Source: CAD feature listing. Evaluate the final solid. Frame: model axes, mm. A direction names the side the tool comes from. Give positions to 0.01 mm unless a question says otherwise; leave off trailing zeros. Order: outer loops, then holes, each group sorted by start corner. A loop starts at its lowest first (then second) coordinate and runs counter-clockwise, first axis right, second up. Notation, with made-up numbers: (66, -23.75) - (103, -23.75) arc R17 cw to (103, 2.25) - close; hole circle Ø10 at (4, 41). An arc over 180 degrees is marked (long way). Use CSV: the item, a comma, the result in double quotes.
```python
from build123d import *

# Parameters (mm, degrees)
BOSS_EXTRUDE1_DEPTH = 10
CUT_EXTRUDE23_DEPTH = 10


with BuildPart() as part:
    # Sketch1 → Boss-Extrude1 (new body)
    with BuildSketch(Plane.XY):
        with BuildLine():
            Line((-50, 60), (50, 60))
            ThreePointArc((50, 60), (57.071067812, 57.071067812), (60, 50))
            Line((60, 50), (60, -50))
            ThreePointArc((60, -50), (57.071067812, -57.071067812), (50, -60))
            Line((50, -60), (-50, -60))
            ThreePointArc((-50, -60), (-57.071067812, -57.071067812), (-60, -50))
            Line((-60, -50), (-60, 50))
            ThreePointArc((-60, 50), (-57.071067812, 57.071067812), (-50, 60))
        make_face()
    extrude(amount=BOSS_EXTRUDE1_DEPTH)

    # Sketch2 → Cut-Extrude23 (cut)
    with BuildSketch(Plane.XY.offset(10)):
        with BuildLine():
            Line((-8.75, 50), (8.75, 50))
            Line((8.75, 50), (8.75, -14.7265625))
            add(Edge.make_bspline(
                [(8.75, -14.7265625), (8.743583975, -15.963662149), (8.731221561, -18.347308928), (8.60745187, -21.778880386), (8.440093422, -24.925119282), (8.199081109, -27.780984325), (7.841111838, -30.346337414), (7.435999316, -32.627578869), (6.989047753, -34.634004111), (6.23403689, -36.879506107), (5.061904404, -39.366144137), (3.293123023, -42.05206658), (1.090424054, -44.385675502), (-1.446357574, -46.412684578), (-4.338596124, -48.017692334), (-7.51966122, -49.177796237), (-10.979383755, -49.870850344), (-13.375676653, -49.956106859), (-14.609375, -50)],
                knots=[0, 0, 0, 0, 1.22248561, 2.355488409, 3.392943897, 4.335991845, 5.186735882, 5.951517034, 6.625683685, 7.215700098, 8.28923535, 9.333114649, 10.380102123, 11.447198135, 12.530158036, 13.633358744, 14.781567393, 16, 16, 16, 16], degree=3))
            add(Edge.make_bspline(
                [(-14.609375, -50), (-15.894776413, -49.960205451), (-18.430089946, -49.88171506), (-22.148388349, -49.2131785), (-25.722137923, -48.141313235), (-29.13284997, -46.591524706), (-32.427252281, -44.650205179), (-35.545554474, -42.242187263), (-38.552862415, -39.442154155), (-40.33561292, -37.293479019), (-41.25, -36.19140625)],
                knots=[0, 0, 0, 0, 0.990984786, 1.954608977, 2.90473533, 3.862451285, 4.837525908, 5.848096122, 6.896271184, 8, 8, 8, 8], degree=3))
            Line((-41.25, -36.19140625), (-28.0078125, -23.9453125))
            add(Edge.make_bspline(
                [(-28.0078125, -23.9453125), (-27.314466509, -24.729291012), (-26.01702976, -26.196325573), (-24.061830829, -28.109374669), (-22.298136041, -29.64628881), (-20.635555645, -30.75487882), (-19.06661841, -31.53631102), (-17.557567552, -32.099198603), (-16.061363785, -32.417824942), (-15.072925956, -32.473022924), (-14.58984375, -32.5)],
                knots=[0, 0, 0, 0, 1.529509877, 2.862124173, 3.996688592, 4.944357383, 5.774364335, 6.554177287, 7.293378699, 8, 8, 8, 8], degree=3))
            add(Edge.make_bspline(
                [(-14.58984375, -32.5), (-14.122273945, -32.475616988), (-13.223290925, -32.428736471), (-11.987154797, -31.907600104), (-10.945012492, -31.089394098), (-10.25892751, -30.148760123), (-9.821709802, -29.187178965), (-9.548527937, -28.257662954), (-9.289277875, -27.143425185), (-9.081572506, -25.845024103), (-8.924629957, -24.345523841), (-8.846405442, -22.663128248), (-8.751274399, -20.78874592), (-8.750439906, -19.479327194), (-8.75, -18.7890625)],
                knots=[0, 0, 0, 0, 1.003927327, 1.930222208, 2.840933547, 3.835773585, 4.407906147, 5.114514582, 5.922289074, 6.876303333, 7.950072246, 9.174518422, 10.510537432, 12, 12, 12, 12], degree=3))
            Line((-8.75, -18.7890625), (-8.75, 50))
        make_face()
    extrude(amount=-CUT_EXTRUDE23_DEPTH, mode=Mode.SUBTRACT)


solid = part.part
```
Item 1: Mould query, pull axis Y, two halves, no side actions, for faces 1 (the flat face through (14, 1, 0)), 2 (the cylindrical face through (-57.15, 56.99, 4.93)), 3 (the flat face through (-34.72, -30.15, 5.07)). Classes: released by +Y, released by -Y, zero draft, split by the parting line, or undercut.
Filled in:
face 1,"zero draft"
face 2,"released by +Y"
face 3,"undercut"
Item 2: First-contact query: pin 1 (1 mm diameter, centred on x = 23, y = -21.5, fed in from -Z). Flat tip, straight axial feed; report the tip coordinate or a pass-through.
Filled in:
pin 1,"stops at z = 0"
Item 3: Set-up query: faces 4 (the flat face through (0, 50, 5)), 5 (the cylindrical face through (-56.99, -57.15, 4.93)). Return all of +Z, -Z, +X, -X, +Y, -Y with unobstructed straight access to the full face (end or side cutting, diameter ignored); none if empty.
Filled in:
face 4,"+Z, -Z"
face 5,"+Z, -Z, -X, -Y"
Item 4: Material intervals for line 1 (X direction, y = 0.5, z = 1); line 2 (X direction, y = -18, z = 1); line 3 (Y direction, x = -30.5, z = 8.75), sorted ascending. Write a range as from..to.
Filled in:
line 1,"x = -60..-8.75, 8.75..60"
line 2,"x = -60..-8.75, 8.72..60"
line 3,"y = -60..-45.76, -26.25..60"
Item 5: Section A-A on y = 47. Return the cut outline in (x, z).
Filled in:
outline,"(-60, 0) - (-8.75, 0) - (-8.75, 10) - (-60, 10) - close; (8.75, 0) - (60, 0) - (60, 10) - (8.75, 10) - close"
